Model file for the job. Use its own axes, mm. Face numbers are marked on the shaded views. A direction names the side the tool comes from. Round coordinates to 2 decimals unless told otherwise and drop trailing zeros. Order: outer loops, then holes, each group sorted by start corner. A loop starts at its lowest first (then second) coordinate and runs counter-clockwise, first axis right, second up. Notation, with made-up numbers: (-18, -9) - (36, -9) arc R6 ccw to (36, -5) - close; hole circle Ø6 at (25, -18.5). An arc over 180 degrees is marked (long way). Put each result on its own line as item: value. Start each with the question number.
Item 1: Which spindle directions (+Z, -Z, +X, -X, +Y, -Y) get a long thin tool onto all of the face, cutting with end or side? Do the marked faces 4, 5, 6 and 7. Say none if no direction does.
Item 2: Saw through at C-C on x = 38.5. List the corners of the cut face in (y, z), plus the area to 3 significant figures.
Item 3: Probe probe 1 along Y at (x, z) = (38.5, -2); probe 2 along X at (y, z) = (20.75, -2.25); probe 3 along Y at (x, z) = (50.5, -2.55). List the from-to ranges inside material, lowest first.
Item 4: Saw through at D-D on z = -7.25. List the corners of the cut face in (x, y), plus the area to 3 significant figures.
Item 5: Pin check, flat tips, straight feed: pin 1 Ø1.6 at (y, z) = (11.5, 4) entering from +X; pin 2 Ø1.4 at (y, z) = (21, 4) entering from +X; pin 3 Ø5 at (y, z) = (7, 5) entering from -X. Stop position of each tip, or through.
Item 6: Saw through at A-A on x = 24.5. List the corners of the cut face in (y, z).
Item 7: Mould opens along X. For the marked faces 1, 2 and 3 say: pulls with the +X half, pulls with the -X half, needs draft (parallel to the pull), parting line crosses it, or undercut.
Item 8: Saw through at B-B on y = 19.25. List the corners of the cut face in (x, z), plus the area to 3 significant figures.
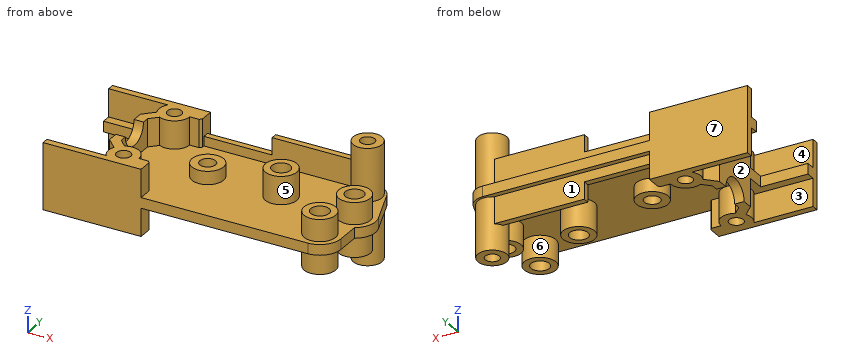
```python
from build123d import *

# Parameters (mm, degrees)
SKETCH2_R           = 1.35
SKETCH2_R_2         = 1.5
SKETCH2_R_3         = 1.75
BOSS_EXTRUDE1_DEPTH = 1
SKETCH3_R           = 3
SKETCH3_R_2         = 1.75
BOSS_EXTRUDE2_DEPTH = 5.15
SKETCH4_R           = 3
SKETCH4_R_2         = 1.75
BOSS_EXTRUDE3_DEPTH = 6.3
SKETCH5_R           = 3
SKETCH5_R_2         = 1.5
BOSS_EXTRUDE4_DEPTH = 3.5
SKETCH6_R           = 2.75
SKETCH6_R_2         = 1.35
BOSS_EXTRUDE5_DEPTH = 11
SKETCH7_R           = 1.35
BOSS_EXTRUDE6_DEPTH = 6.3
BOSS_EXTRUDE7_DEPTH = 1.2
SKETCH9_R           = 1.35
CUT_EXTRUDE1_DEPTH  = 23
CUT_EXTRUDE2_REACH  = 49.5
CHAMFER2_SIZE       = 0.4


with BuildPart() as part:
    # Sketch2 → Boss-Extrude1 (new body, symmetric)
    with BuildSketch(Plane.XY):
        with BuildLine():
            Line((0, 0), (50.5, 0))
            ThreePointArc((50.5, 0), (53.328427125, 1.171572875), (54.5, 4))
            Line((54.5, 4), (54.5, 8.535898385))
            ThreePointArc((54.5, 8.535898385), (56.259762135, 10.634647047), (56.256781243, 13.373533652))
            Line((56.256781243, 13.373533652), (53.505424994, 20.898826922))
            ThreePointArc((53.505424994, 20.898826922), (52.33354218, 22.4226176), (50.5, 23))
            Line((50.5, 23), (0, 23))
            Line((0, 23), (0, 20))
            Line((0, 20), (9, 20))
            Line((9, 20), (9, 3))
            Line((9, 3), (0, 3))
            Line((0, 3), (0, 0))
        make_face()
        with Locations((13.6, 3.1)):
            Circle(SKETCH2_R, mode=Mode.SUBTRACT)
        with Locations((24.5, 12)):
            Circle(SKETCH2_R_2, mode=Mode.SUBTRACT)
        with Locations((38.5, 12)):
            Circle(SKETCH2_R_3, mode=Mode.SUBTRACT)
        with Locations((52.5, 12)):
            Circle(SKETCH2_R_3, mode=Mode.SUBTRACT)
        with Locations((50.5, 4)):
            Circle(SKETCH2_R_3, mode=Mode.SUBTRACT)
        with Locations((50.5, 19.8)):
            Circle(SKETCH2_R, mode=Mode.SUBTRACT)
        with Locations((13.6, 19.9)):
            Circle(SKETCH2_R, mode=Mode.SUBTRACT)
    extrude(amount=BOSS_EXTRUDE1_DEPTH, both=True)

    # Sketch3 → Boss-Extrude2 (add, symmetric)
    with BuildSketch(Plane.XY):
        with Locations((50.5, 4)):
            Circle(SKETCH3_R)
        with Locations((50.5, 4)):
            Circle(SKETCH3_R_2, mode=Mode.SUBTRACT)
        with Locations((52.5, 12)):
            Circle(SKETCH3_R)
        with Locations((52.5, 12)):
            Circle(SKETCH3_R_2, mode=Mode.SUBTRACT)
    extrude(amount=BOSS_EXTRUDE2_DEPTH, both=True)

    # Sketch4 → Boss-Extrude3 (add, symmetric)
    with BuildSketch(Plane.XY):
        with Locations((38.5, 12)):
            Circle(SKETCH4_R)
        with Locations((38.5, 12)):
            Circle(SKETCH4_R_2, mode=Mode.SUBTRACT)
    extrude(amount=BOSS_EXTRUDE3_DEPTH, both=True)

    # Sketch5 → Boss-Extrude4 (add, symmetric)
    with BuildSketch(Plane.XY):
        with Locations((24.5, 12)):
            Circle(SKETCH5_R)
        with Locations((24.5, 12)):
            Circle(SKETCH5_R_2, mode=Mode.SUBTRACT)
    extrude(amount=BOSS_EXTRUDE4_DEPTH, both=True)

    # Sketch6 → Boss-Extrude5 (add, symmetric)
    with BuildSketch(Plane.XY):
        with Locations((50.5, 19.8)):
            Circle(SKETCH6_R)
        with Locations((50.5, 19.8)):
            Circle(SKETCH6_R_2, mode=Mode.SUBTRACT)
    extrude(amount=BOSS_EXTRUDE5_DEPTH, both=True)

    # Sketch7 → Boss-Extrude6 (add, symmetric)
    with BuildSketch(Plane.XY):
        with BuildLine():
            Line((0, 23), (18.7, 23))
            Line((18.7, 23), (18.7, 19.9))
            Line((18.7, 19.9), (16.5, 19.9))
            ThreePointArc((16.5, 19.9), (15.108348306, 17.423129921), (12.269044559, 17.323460147))
            Line((12.269044559, 17.323460147), (10.8, 15.854415588))
            Line((10.8, 15.854415588), (10.8, 11.5))
            Line((10.8, 11.5), (10.8, 7.145584412))
            Line((10.8, 7.145584412), (12.269044559, 5.676539853))
            ThreePointArc((12.269044559, 5.676539853), (15.108348306, 5.576870079), (16.5, 3.1))
            Line((16.5, 3.1), (18.7, 3.1))
            Line((18.7, 3.1), (18.7, 0))
            Line((18.7, 0), (0, 0))
            Line((0, 0), (0, 1.3))
            Line((0, 1.3), (11.3262366, 1.3))
            ThreePointArc((11.3262366, 1.3), (10.715483905, 2.800722707), (11.005134966, 4.394865034))
            Line((11.005134966, 4.394865034), (9, 6.4))
            Line((9, 6.4), (9, 11.5))
            Line((9, 11.5), (9, 16.6))
            Line((9, 16.6), (11.005134966, 18.605134966))
            ThreePointArc((11.005134966, 18.605134966), (10.715483905, 20.199277293), (11.3262366, 21.7))
            Line((11.3262366, 21.7), (0, 21.7))
            Line((0, 21.7), (0, 23))
        make_face()
        with Locations((13.6, 3.1)):
            Circle(SKETCH7_R, mode=Mode.SUBTRACT)
        with Locations((13.6, 19.9)):
            Circle(SKETCH7_R, mode=Mode.SUBTRACT)
    extrude(amount=BOSS_EXTRUDE6_DEPTH, both=True)

    # Sketch8 → Boss-Extrude7 (add)
    with BuildSketch(Plane(origin=(0, 22, 0), x_dir=(-1, 0, 0), z_dir=(0, 1, 0))):
        Polygon((-18.7, -2.8), (-18.7, 2.8), (-31.7, 2.8), (-31.7, 6.05), (-50.5, 6.05), (-50.5, -6.05), (-31.7, -6.05), (-31.7, -2.8), align=None)
    extrude(amount=-BOSS_EXTRUDE7_DEPTH)

    # Sketch9 → Cut-Extrude1 (cut, through all)
    with BuildSketch(Plane(origin=(0, 0, -11), x_dir=(-1, 0, 0), z_dir=(0, 0, -1))):
        with Locations((-50.5, 19.8)):
            Circle(SKETCH9_R)
    extrude(amount=-CUT_EXTRUDE1_DEPTH, mode=Mode.SUBTRACT)

    # Sketch10 → Cut-Extrude2 (cut, up to next)
    with BuildSketch(Plane.ZY.offset(-9), mode=Mode.PRIVATE) as cut_extrude2_sk1:
        with BuildLine():
            Line((-6.3, 14.5), (-6.3, 8.5))
            ThreePointArc((-6.3, 8.5), (-3.3, 11.5), (-6.3, 14.5))
        make_face()
    cut_extrude2_tool1 = extrude(cut_extrude2_sk1.sketch, amount=-CUT_EXTRUDE2_REACH, mode=Mode.PRIVATE) & part.part
    add(cut_extrude2_tool1.solids().sort_by_distance((9, 11.5, -5.02676))[0], mode=Mode.SUBTRACT)
    # Sketch10 → Cut-Extrude2 (cut, up to next)
    with BuildSketch(Plane.ZY.offset(-9), mode=Mode.PRIVATE) as cut_extrude2_sk2:
        with BuildLine():
            Line((6.3, 8.5), (6.3, 14.5))
            ThreePointArc((6.3, 14.5), (3.3, 11.5), (6.3, 8.5))
        make_face()
    cut_extrude2_tool2 = extrude(cut_extrude2_sk2.sketch, amount=-CUT_EXTRUDE2_REACH, mode=Mode.PRIVATE) & part.part
    add(cut_extrude2_tool2.solids().sort_by_distance((9, 11.5, 5.02676))[0], mode=Mode.SUBTRACT)

    # Chamfer2
    chamfer2_edges = [part.edges().sort_by_distance(p)[0] for p in [
        (18.7, 3.1, -3.65),
        (18.7, 19.9, -3.65),
        (18.7, 3.1, 3.65),
        (18.7, 19.9, 3.65),
    ]]
    chamfer(chamfer2_edges, length=CHAMFER2_SIZE)


solid = part.part
```
Results found:
1. face 4: +Z, -X
1. face 5: +Z
1. face 6: -Z
1. face 7: +Z, -Z, +X, -X, +Y
2. outline: (0, -1) - (9, -1) - (9, -6.3) - (10.25, -6.3) - (10.25, 6.3) - (9, 6.3) - (9, 1) - (0, 1) - close; (13.75, -6.3) - (15, -6.3) - (15, -1) - (20.8, -1) - (20.8, -6.05) - (22, -6.05) - (22, -1) - (23, -1) - (23, 1) - (22, 1) - (22, 6.05) - (20.8, 6.05) - (20.8, 1) - (15, 1) - (15, 6.3) - (13.75, 6.3) - close
2. area: 77.6 mm²
3. probe 1: y = 9 to 10.25, 13.75 to 15, 20.8 to 22
3. probe 2: x = 10.83 to 12.55, 14.65 to 18.7, 47.92 to 49.54, 51.46 to 53.08
3. probe 3: y = 1 to 2.25, 5.75 to 7, 9.76 to 14.24, 17.05 to 18.45, 21.15 to 22.55
4. outline: circle Ø5.5 at (50.5, 19.8); hole circle Ø2.7 at (50.5, 19.8)
4. area: 18.0 mm²
5. pin 1: stops at x = 55.5
5. pin 2: stops at x = 53.2
5. pin 3: stops at x = 9
6. outline: (0, -1) - (9, -1) - (9, -3.5) - (10.5, -3.5) - (10.5, 3.5) - (9, 3.5) - (9, 1) - (0, 1) - close; (13.5, -3.5) - (15, -3.5) - (15, -1) - (20.8, -1) - (20.8, -2.8) - (22, -2.8) - (22, -1) - (23, -1) - (23, 1) - (22, 1) - (22, 2.8) - (20.8, 2.8) - (20.8, 1) - (15, 1) - (15, 3.5) - (13.5, 3.5) - close
7. face 1: undercut
7. face 2: pulls with the -X half
7. face 3: needs draft
8. outline: (9, -1) - (10.77, -1) - (10.77, -6.3) - (12.42, -6.3) - (12.42, 6.3) - (10.77, 6.3) - (10.77, 1) - (9, 1) - close; (14.78, -6.3) - (16.43, -6.3) - (16.43, -1) - (47.81, -1) - (47.81, -11) - (49.27, -11) - (49.27, 11) - (47.81, 11) - (47.81, 1) - (16.43, 1) - (16.43, 6.3) - (14.78, 6.3) - close; (51.73, -11) - (53.19, -11) - (53.19, -1) - (54.11, -1) - (54.11, 1) - (53.19, 1) - (53.19, 11) - (51.73, 11) - close
8. area: 174 mm²
